from build123d import *

# Parameters (mm, degrees)
F0_W     = 10
F0_H     = 10
F0_W_2   = 8
F0_H_2   = 8
F1_DEPTH = 55
F2_R     = 1.5
F3_DEPTH = 25
F4_R     = 2.5
F5_DEPTH = 25


with BuildPart() as f1:
    # F0 (on Front) → F1 (new body)
    with BuildSketch(Plane.XZ):
        Rectangle(F0_W, F0_H)
        Rectangle(F0_W_2, F0_H_2, mode=Mode.SUBTRACT)
    extrude(amount=F1_DEPTH)

    # F2 (on face) → F3 (cut)
    with BuildSketch(Plane.YZ.offset(5)):
        with Locations((-50, 0)):
            Circle(F2_R)
        with Locations((-5, 0)):
            Circle(F2_R)
    extrude(amount=-F3_DEPTH, mode=Mode.SUBTRACT)

    # F4 (on face) → F5 (cut)
    with BuildSketch(Plane.XY.offset(5)):
        with Locations((-1, -40.5)):
            Circle(F4_R)
        with Locations((-1, -14.5)):
            Circle(F4_R)
    extrude(amount=-F5_DEPTH, mode=Mode.SUBTRACT)


solid = f1.part
Model file for the job. Use its own axes, mm. A direction names the side the tool comes from. Give positions to 0.01 mm unless a question says otherwise; leave off trailing zeros. Order: outer loops, then holes, each group sorted by start corner. A loop starts at its lowest first (then second) coordinate and runs counter-clockwise, first axis right, second up. Notation, with made-up numbers: (-28, -32) -> (-23, -32) arc R22 cw to (-23, -10) -> close; hole circle Ø7 at (79.25, -8.5). An arc over 180 degrees is marked (long way). Use CSV: the item, a comma, the result in double quotes.
1. Band-saw the part on D-D, the plane z = 0. Give the cut face in (x, y).
Outcome:
outline,"(-5, -55) -> (-4, -55) -> (-4, -51.5) -> (-5, -51.5) -> close; (-5, -48.5) -> (-4, -48.5) -> (-4, -6.5) -> (-5, -6.5) -> close; (-5, -3.5) -> (-4, -3.5) -> (-4, 0) -> (-5, 0) -> close; (4, -55) -> (5, -55) -> (5, -51.5) -> (4, -51.5) -> close; (4, -48.5) -> (5, -48.5) -> (5, -6.5) -> (4, -6.5) -> close; (4, -3.5) -> (5, -3.5) -> (5, 0) -> (4, 0) -> close"
2. Drop a flat-ended pin along its axis: pin 1 (2.5 mm diameter, centred on y = -5, z = 0, fed in from -X). Give the stop position or say it passes through.
Outcome:
pin 1,"through"
3. 3-axis set-ups, long thin cutter, end or side, ignore diameter. For faces 5 (the cylindrical face through (-1.54, -42.94, 4.51)), 6 (the flat face through (0, -27, 4)): which of +Z, -Z, +X, -X, +Y, -Y reach the whole face in a straight line?
Outcome:
face 5,"+Z, -Z"
face 6,"+Y, -Y"
4. Drill centre lines: line 1 along Y through (x, z) = (-1, -4.8); line 2 along X through (y, z) = (-48.5, 2); line 3 along Z through (x, y) = (4.3, -5). Where is each one in solid material? Low to high. Write a range as from..to.
Outcome:
line 1,"-55..-43, -38..-17, -12..0"
line 2,"-5..-4, 4..5"
line 3,"-5..-1.5, 1.5..5"
5. Band-saw the part on A-A, the plane x = 1. Give the cut face in (y, z), then the cut area to 3 significant figures.
Outcome:
outline,"(-55, -5) -> (-42, -5) -> (-42, -4) -> (-55, -4) -> close; (-55, 4) -> (-42, 4) -> (-42, 5) -> (-55, 5) -> close; (-39, -5) -> (-16, -5) -> (-16, -4) -> (-39, -4) -> close; (-39, 4) -> (-16, 4) -> (-16, 5) -> (-39, 5) -> close; (-13, -5) -> (0, -5) -> (0, -4) -> (-13, -4) -> close; (-13, 4) -> (0, 4) -> (0, 5) -> (-13, 5) -> close"
area,"98.0 mm²"
6. Mould opens along X. For faces 1 (the flat face through (4, -27, 0)), 2 (the flat face through (5, -27, 0)), 3 (the cylindrical face through (-1.54, -16.94, 4.51)), 4 (the flat face through (-4.5, 0, 0.1)) say: +X half, -X half, draft (parallel to the pull), parting line (faces both ways), or undercut.
Outcome:
face 1,"undercut"
face 2,"+X half"
face 3,"undercut"
face 4,"draft"
7. Band-saw the part on C-C, the plane z = 3.25. Give the cut face in (x, y), then the cut area to 3 significant figures.
Outcome:
outline,"(-5, -55) -> (-4, -55) -> (-4, 0) -> (-5, 0) -> close; (4, -55) -> (5, -55) -> (5, 0) -> (4, 0) -> close"
area,"110 mm²"
8. Band-saw the part on B-B, the plane y = -50. Give the cut face in (x, z), then the cut area to 3 significant figures.
Outcome:
outline,"(-5, -5) -> (5, -5) -> (5, -1.5) -> (4, -1.5) -> (4, -4) -> (-4, -4) -> (-4, -1.5) -> (-5, -1.5) -> close; (-5, 1.5) -> (-4, 1.5) -> (-4, 4) -> (4, 4) -> (4, 1.5) -> (5, 1.5) -> (5, 5) -> (-5, 5) -> close"
area,"30.0 mm²"
